Autodesk Inventor part; units mm, degrees
ref_plane "YZ Plane" through (0, 0, 0) normal (1, 0, 0) x (0, 1, 0)
ref_plane "XZ Plane" through (0, 0, 0) normal (0, 1, 0) x (-1, 0, 0)
ref_plane "XY Plane" through (0, 0, 0) normal (0, 0, 1) x (1, 0, 0)
sketch "Sketch2" plane through (0, 0, 0) normal (1, 0, 0) x (0, 1, 0)
  circle A0 centre (0, 0) radius 1.25
  dimension "d8" = 2.5
extrude "Extrusion1" add sketch "Sketch2" along normal blind 14
sketch "Sketch6" plane through (0, 0, 0) normal (0, 0, 1) x (1, 0, 0)
  line L0 (14, -1.25) -> (14, 1.25)
  line L1 (14, 0) -> (14, 0.125)
  line L2 (14, 0.125) -> (15.875, 0.125)
  line L3 (16, 0) -> (16, -15.875)
  line L4 (14, 0) -> (15.875, 0)
  line L5 (15.875, 0) -> (15.875, -15.875)
  line L6 (15.875, -15.875) -> (16, -15.875)
  line L7 (15.875, 0) -> (16, 0)
  line L8 (17.9417, 0) -> (15.75, 0)
  arc A0 (15.875, -0.125) -> (15.75, 0) centre (15.75, -0.125) ccw
  line L9 (15.75, 0) -> (16, 0)
  line L10 (0, 0) -> (0, 0.125)
  line L11 (0, 0.125) -> (-1.875, 0.125)
  line L12 (-2, 0) -> (-2, -15.875)
  line L13 (-2, -15.875) -> (-1.875, -15.875)
  line L14 (-1.875, -15.875) -> (-1.875, -0.125)
  line L15 (-1.75, 0) -> (0, 0)
  arc A1 (-1.875, 0.125) -> (-2, 0) centre (-1.875, 0) ccw
  arc A2 (-1.75, 0) -> (-1.875, -0.125) centre (-1.75, -0.125) ccw
  line L16 (-1.75, 0) -> (-2, 0)
  line L17 (-1.875, -0.125) -> (-1.875, 0)
  arc A3 (16, 0) -> (15.875, 0.125) centre (15.875, 0) ccw
  point P0 (16, 0.125)
  point P1 (18.875, 0.125)
  point P2 (-2, 0.125)
  point P3 (-1.875, 0)
  dimension "d16" = 0.125
  dimension "d17" = 2
  dimension "d18" = 16
  dimension "d19" = 1.875
  dimension "d26" = 0.125
  dimension "d27" = 2
  dimension "d28" = 0.125
  dimension "d29" = 0.125
  dimension "d30" = 0.125
  dimension "d33" = 0.125
  dimension "d35" = 16
revolve "Revolution2" add sketch "Sketch6" angle 360 about axis through (14, 0, 0) along (1, 0, 0) contours L0 L2 A3 L7 L4
revolve "Revolution3" add sketch "Sketch6" angle 360 about axis through (15.875, 0, 0) along (0, -1, 0) contours L7 L3 L6 L5
revolve "Revolution4" add sketch "Sketch6" angle 360 about axis through (-1.75, 0, 0) along (1, 0, 0) contours L15 L16 A1 L11 L10
revolve "Revolution5" add sketch "Sketch6" angle 360 about axis through (-1.875, -15.875, 0) along (0, 1, 0) contours L14 L13 L12 L16 L17
equation "\"d35\" = d18"
properties part number "Reed Switch Frontal" material "Aluminum 6061"
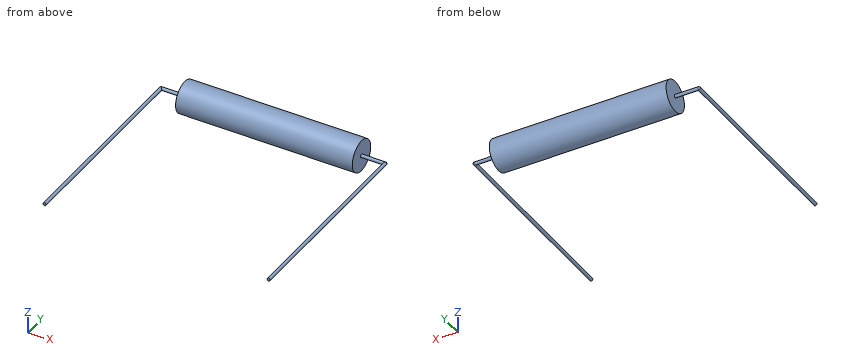
Part model, mm, in its own coordinate system. Round coordinates to 2 decimals unless told otherwise and drop trailing zeros. Write each loop counter-clockwise with the first axis right and the second up, starting at its lowest first coordinate (ties: lowest second). Pieces come first, ordered by that corner, then holes. Notation, with made-up numbers: M 48,50.25 L 55,50.25 A23 ccw 55,61.25 Z; hole C -37.5,32.5 d4. An arc over 180 degrees is marked long. One line per question, with ' | ' between items.
(1) Saw through at B-B on x = 0.5. Write the cut outline in (y, z), then the cut area to 3 significant figures.
Answer key:
outline: C 0,0 d2.5 | area: 4.91 mm^2
(2) Pin check, flat tips, straight feed: pin 1 (0.8 mm diameter, centred on y = 0.5, z = -0.5, fed in from +X); pin 2 (1.5 mm diameter, centred on y = -13.5, z = -0.5, fed in from +X). Stop position of each tip, or through.
Answer key:
pin 1: stops at x = 14 | pin 2: stops at x = 16
(3) Saw through at A-A on y = -13. Write the cut outline in (x, z) (3 decimals).
Answer key:
outline: C -1.875,0 d0.25; C 15.875,0 d0.25
(4) Probe line 1 along X through (y, z) = (0.5, 1); line 2 along Y through (x, z) = (11, -0.1); line 3 along Y through (x, z) = (4.75, 0.7). List the from-to ranges inside material, lowest first.
Answer key:
line 1: x = 0 to 14 | line 2: y = -1.25 to 1.25 | line 3: y = -1.04 to 1.04
(5) Saw through at C-C on z = -0.7. Write the cut outline in (x, y), then the cut area to 3 significant figures.
Answer key:
outline: M 0,-1.04 L 14,-1.04 L 14,1.04 L 0,1.04 Z | area: 29.0 mm^2
